from build123d import *

# Parameters (mm, degrees)
SKETCH011_R           = 10
PAD007_DEPTH          = 14.5
CHAMFER008_SIZE       = 0.4
SKETCH012_R           = 0.75
POCKET_DEPTH          = 3.501
SKETCH013_R           = 9
POCKET001_DEPTH       = 12.25
POCKET002_DEPTH       = 78.56986
POLARPATTERN002_COUNT = 8
CHAMFER004014008_SIZE = 2.24
CHAMFER004014009_SIZE = 0.5
CHAMFER004014010_SIZE = 0.45


with BuildPart() as part:
    # Sketch011 (on DatumPlane) → Pad007 (new body)
    with BuildSketch(Plane.XY):
        Circle(SKETCH011_R)
    extrude(amount=PAD007_DEPTH)

    # Chamfer008
    chamfer008_edges = [part.edges().sort_by_distance(p)[0] for p in [
        (-10, 0, 14.5),
    ]]
    chamfer(chamfer008_edges, length=CHAMFER008_SIZE)

    # Sketch012 (on DatumPlane) → Pocket (cut, through all)
    with BuildSketch(Plane.XY.offset(11)):
        Circle(SKETCH012_R)
    extrude(amount=POCKET_DEPTH, mode=Mode.SUBTRACT)

    # Sketch013 (on DatumPlane) → Pocket001 (cut)
    with BuildSketch(Plane.XY):
        Circle(SKETCH013_R)
    extrude(amount=POCKET001_DEPTH, mode=Mode.SUBTRACT)

    # Sketch019 (on DatumPlane) → Pocket002 (cut, through all)
    with BuildSketch(Plane.XY.offset(15)):
        with BuildLine():
            ThreePointArc((8.467655, -0.740824), (8.5, 0), (8.467655, 0.740824))
            Line((5.479071, 0.479357), (8.467655, 0.740824))
            ThreePointArc((5.479071, -0.479357), (5.5, 0), (5.479071, 0.479357))
            Line((5.479071, -0.479357), (8.467655, -0.740824))
        make_face()
    pocket002 = extrude(amount=-POCKET002_DEPTH, mode=Mode.SUBTRACT)

    # PolarPattern002: Pocket002 ×8 about axis
    polarpattern002_axis = Axis((0, 0, 15), (0, 0, 1))
    for i in range(1, POLARPATTERN002_COUNT):
        add(pocket002.rotate(polarpattern002_axis, i * 360 / POLARPATTERN002_COUNT), mode=Mode.SUBTRACT)

    # Chamfer004014008
    chamfer004014008_edges = [part.edges().sort_by_distance(p)[0] for p in [
        (-5.362311, -4.499513, 12.25),
        (-6.973363, 0.61009, 12.25),
        (-4.499513, 5.362311, 12.25),
        (0.61009, 6.973363, 12.25),
        (5.362311, 4.499513, 12.25),
        (6.973363, -0.61009, 12.25),
        (4.499513, -5.362311, 12.25),
        (-0.61009, -6.973363, 12.25),
        (-6.973363, -0.61009, 14.5),
        (-5.362311, 4.499513, 14.5),
        (-0.61009, 6.973363, 14.5),
        (4.499513, 5.362311, 14.5),
        (6.973363, 0.61009, 14.5),
        (5.362311, -4.499513, 14.5),
        (0.61009, -6.973363, 14.5),
        (-4.499513, -5.362311, 14.5),
    ]]
    chamfer(chamfer004014008_edges, length=CHAMFER004014008_SIZE)

    # Chamfer004014009
    chamfer004014009_edges = [part.edges().sort_by_distance(p)[0] for p in [
        (-9, 0, 0),
    ]]
    chamfer(chamfer004014009_edges, length=CHAMFER004014009_SIZE)

    # Chamfer004014010
    chamfer004014010_edges = [part.edges().sort_by_distance(p)[0] for p in [
        (-9, 0, 12.25),
    ]]
    chamfer(chamfer004014010_edges, length=CHAMFER004014010_SIZE)


with BuildPart() as part_1:
    # Body002002003003 placement: moved
    add(part.part.moved(Location((0, 0, 2))))


solid = part_1.part
Can you work these out from the model? Positions are in its coordinate system, mm. A direction names the side the tool comes from. Give positions to 0.01 mm unless a question says otherwise; leave off trailing zeros. Write each loop counter-clockwise with the first axis right and the second up, starting at its lowest first coordinate (ties: lowest second). Pieces come first, ordered by that corner, then holes. Notation, with made-up numbers: (30, 4) -> (83, 4) arc R25 cw to (83, 36) -> close; hole circle Ø10 at (73, 58). An arc over 180 degrees is marked (long way). Answer as a JSON object with one key per item and string values. Group by question number.
Item 1: Suppose I cut it at A-A (y = 0). Please give me the cut outline in (x, z).
Item 2: For faces 1 (the face through (-6.61, 1.72, 15.35)), 2 (the face through (-3.485, -5.871, 15.364)), 3 (the face through (-6.04, -5.98, 15.39)), 4 (the face through (-2.17, -9.76, 8.95)), which set-ups out of +Z, -Z, +X, -X, +Y, -Y let a thin tool reach every point of the face, with its end or its side?
Item 3: Suppose I cut it at D-D (z = 9). Please give me the cut outline in (x, y), plus the area to 3 significant figures.
Item 4: We'd pull the mould along Z, two halves only. Please class faces 5 (the face through (-5.871, 3.485, 15.364)), 6 (the face through (-1.172, 8.923, 8.071)), 7 (the face through (-5.891, -3.461, 15.354)): +Z half, -Z half, draft (parallel to the pull), parting line (faces both ways), or undercut.
Item 5: I'm going to push flat-ended pins straight in: P1, Ø5, axis at x = -5, z = 12.5, coming from the -Y side; P2, Ø2.5, axis at x = 0, y = 0, coming from the +Z side; P3, Ø4, axis at x = -7, y = -2, coming from the -Z side; P4, Ø1.5, axis at x = 1, y = 0.5, coming from the -Z side. Where does each tip first touch, or does it pass through?
Item 6: Please list where these lines run through material, in increasing order: line 1 (Y direction, x = 0, z = 15.8); line 2 (Y direction, x = 0, z = 8.75); line 3 (Y direction, x = -1.25, z = 15.5). Write a range as [from, to].
Item 7: Suppose I cut it at C-C (z = 14.75). State how many separate pieces and enclosed holes the cut face has, plus the area to 3 significant figures.
Findings:
{
 "1": {"outline": "(-10, 2) -> (-9.5, 2) -> (-9, 2.5) -> (-9, 13.8) -> (-8.55, 14.25) -> (-8.5, 14.25) -> (-8.5, 16.5) -> (-9.6, 16.5) -> (-10, 16.1) -> close; (-5.5, 14.25) -> (-0.75, 14.25) -> (-0.75, 16.5) -> (-5.5, 16.5) -> close; (0.75, 14.25) -> (5.5, 14.25) -> (5.5, 16.5) -> (0.75, 16.5) -> close; (8.5, 14.25) -> (8.55, 14.25) -> (9, 13.8) -> (9, 2.5) -> (9.5, 2) -> (10, 2) -> (10, 16.1) -> (9.6, 16.5) -> (8.5, 16.5) -> close"},
 "2": {"face 1": "-Z", "face 2": "+Z", "face 3": "none", "face 4": "+Z, -Z"},
 "3": {"outline": "circle Ø20 at (0, 0); hole circle Ø18 at (0, 0)", "area": "59.7 mm²"},
 "4": {"face 5": "+Z half", "face 6": "draft", "face 7": "-Z half"},
 "5": {"P1": "stops at y = -9.68", "P2": "stops at z = 16.5", "P3": "stops at z = 2.22", "P4": "stops at z = 14.25"},
 "6": {"line 1": "y = [-10, -8.5], [-5.5, -0.75], [0.75, 5.5], [8.5, 10]", "line 2": "y = [-10, -9], [9, 10]", "line 3": "y = [-9.92, -8.41], [-5.36, 5.36], [8.41, 9.92]"},
 "7": {"separate pieces": "1", "enclosed holes": "9", "area": "229 mm²"}
}
